Geometry check sheet. Reference: the model listing, model coordinates, mm. A direction names the side the tool comes from. Give positions to 0.01 mm unless a question says otherwise; leave off trailing zeros. Loops run counter-clockwise (first coordinate to the right, second up) from the corner with the lowest first, then second, coordinate; pieces in that order, holes last.
1. Go/stop test with flat-tipped pins: pin 1 Ø3 at (x, z) = (-36.5, 41) entering from -Y; pin 2 Ø10 at (y, z) = (23.5, 9) entering from -X; pin 3 Ø5.5 at (x, y) = (-39.5, 32) entering from +Z; pin 4 Ø2.5 at (x, z) = (39.5, 3.5) entering from +Y. Record where each tip stops, or that it passes through.
2. Cross-section at B-B, the plane y = 28. Record the cut outline in (x, z), plus the area to 3 significant figures.
3. Cross-section at C-C, the plane x = -20. Record the cut outline in (y, z).
4. Tool access check on faces 1 (the flat face through (-41.2, 22.3, 5)), 2 (the flat face through (0, 17, 5)), 3 (the flat face through (-43, 26, 25)), 4 (the flat face through (-39, 14.731, 25)). Record the directions out of +Z, -Z, +X, -X, +Y, -Y that give a thin tool (end or side, any length) a straight path to the whole face; none if there is none.
5. Release check for a two-part mould opening along Z. For faces 5 (the flat face through (-41.2, 25.6, 15)), 6 (the flat face through (0, 26, 50)), 7 (the flat face through (41, 29, 2)), 8 (the flat face through (0, 17, 0)) record: +Z half, -Z half, draft (parallel to the pull), parting line (faces both ways), or undercut.
6. Cross-section at D-D, the plane z = 3. Record the cut outline in (x, y), plus the area to 3 significant figures.
7. Material ranges on L1, parallel to Z at x = -36.5, y = 12.3; L2, parallel to X at y = 21, z = 3; L3, parallel to Z at x = -42, y = 29, recorded low to high.
8. Cross-section at A-A, the plane z = 25. Record the cut outline in (x, y).
from build123d import *

# Parameters (mm, degrees)
F1_DEPTH    = 50
F3_DEPTH    = 15
F5_DEPTH    = 15
F6_R        = 2.5
F7_DEPTH    = 93.001
F8_T1_DEPTH = 57.6539038248
F9_DEPTH    = 5
F10_R       = 2
F11_DEPTH   = 33


# Not quite as in the source:
# - a fillet or chamfer that OpenCascade refuses, or shapes differently, is made with other operations: its cross-section is extruded or revolved along the edge and cut away or added


with BuildPart() as f1:
    # F0 (on Top) → F1 (new body)
    with BuildSketch(Plane.XY):
        with BuildLine():
            ThreePointArc((-43, 8.7560448021), (-46.7056429154, 4.5424231597), (-50, 0))
            Line((-50, 0), (-47.5900705485, 0))
            ThreePointArc((-47.5900705485, 0), (-26.8784989109, 18.3696900801), (0, 25))
            ThreePointArc((0, 25), (26.8784989109, 18.3696900801), (47.5900705485, 0))
            Line((47.5900705485, 0), (50, 0))
            ThreePointArc((50, 0), (46.7056429154, 4.5424231597), (43, 8.7560448021))
            Line((43, 8.7560448021), (43, 43))
            Line((43, 43), (41, 43))
            Line((41, 43), (41, 14.7306729384))
            Line((41, 14.7306729384), (36.2875219066, 14.7306729384))
            ThreePointArc((36.2875219066, 14.7306729384), (0, 27), (-36.2875219066, 14.7306729384))
            Line((-36.2875219066, 14.7306729384), (-41, 14.7306729384))
            Line((-41, 14.7306729384), (-41, 43))
            Line((-41, 43), (-43, 43))
            Line((-43, 43), (-43, 8.7560448021))
        make_face()
    extrude(amount=F1_DEPTH)

    # F2 (on face) → F3 (cut)
    with BuildSketch(Plane.XY.offset(50)):
        Polygon((-43, 8.7560448021), (-36.2875219066, 14.7306729384), (-41, 14.7306729384), (-41, 43), (-43, 43), align=None)
        Polygon((41, 43), (41, 14.7306729384), (36.2875219066, 14.7306729384), (43, 8.7560448021), (43, 43), align=None)
    extrude(amount=-F3_DEPTH, mode=Mode.SUBTRACT)

    # F4 (on face) → F5 (cut)
    with BuildSketch(Plane(origin=(0, 0, 0), x_dir=(1, 0, 0), z_dir=(0, 0, -1))):
        Polygon((-36.2875219066, -14.7306729384), (-43, -8.7560448021), (-43, -43), (-41, -43), (-41, -14.7306729384), align=None)
        Polygon((43, -8.7560448021), (36.2875219066, -14.7306729384), (41, -14.7306729384), (41, -43), (43, -43), align=None)
    extrude(amount=-F5_DEPTH, mode=Mode.SUBTRACT)

    # F6 (on face) → F7 (cut, through all)
    with BuildSketch(Plane(origin=(-43, 0, 0), x_dir=(0, -1, 0), z_dir=(-1, 0, 0))):
        with Locations((-29.5, 25)):
            Circle(F6_R)
    extrude(amount=-F7_DEPTH, mode=Mode.SUBTRACT)

    # F8: chamfer of 1.5 on 2 edges, made by hand

    # F8_s2 → F8_t1 (cut)
    with BuildSketch(Plane.XY.offset(-3.8269519124)):
        with BuildLine():
            Line((-49.1206089535, -0.027238599), (-46.7036689522, 1.2042065191))
            Line((-46.7036689522, 1.2042065191), (-46.6793989906, 1.186572207))
            ThreePointArc((-46.6793989906, 1.186572207), (-47.1374385844, 0.5954223102), (-47.565368237, -0.0170233899))
            Line((-47.565368237, -0.0170233899), (-47.5900705485, -0.03))
            ThreePointArc((-47.5900705485, -0.03), (-48.355339751, -0.03), (-49.1206089535, -0.057238599))
            Line((-49.1206089535, -0.057238599), (-49.1206089535, -0.027238599))
        make_face()
        with BuildLine():
            Line((46.7036689522, 1.2042065191), (49.1206089535, -0.027238599))
            Line((49.1206089535, -0.027238599), (49.1206089535, -0.057238599))
            ThreePointArc((49.1206089535, -0.057238599), (48.355339751, -0.03), (47.5900705485, -0.03))
            Line((47.5900705485, -0.03), (47.565368237, -0.0170233899))
            ThreePointArc((47.565368237, -0.0170233899), (47.1374385844, 0.5954223102), (46.6793989906, 1.186572207))
            Line((46.6793989906, 1.186572207), (46.7036689522, 1.2042065191))
        make_face()
    extrude(amount=F8_T1_DEPTH, mode=Mode.SUBTRACT)

    # F0 (on Top) → F9 (join)
    with BuildSketch(Plane.XY):
        with BuildLine():
            ThreePointArc((-43, 8.7560448021), (-46.7056429154, 4.5424231597), (-50, 0))
            Line((-50, 0), (-47.5900705485, 0))
            ThreePointArc((-47.5900705485, 0), (-26.8784989109, 18.3696900801), (0, 25))
            ThreePointArc((0, 25), (26.8784989109, 18.3696900801), (47.5900705485, 0))
            Line((47.5900705485, 0), (50, 0))
            ThreePointArc((50, 0), (46.7056429154, 4.5424231597), (43, 8.7560448021))
            Line((43, 8.7560448021), (43, 43))
            Line((43, 43), (41, 43))
            Line((41, 43), (41, 14.7306729384))
            Line((41, 14.7306729384), (36.2875219066, 14.7306729384))
            ThreePointArc((36.2875219066, 14.7306729384), (0, 27), (-36.2875219066, 14.7306729384))
            Line((-36.2875219066, 14.7306729384), (-41, 14.7306729384))
            Line((-41, 14.7306729384), (-41, 43))
            Line((-41, 43), (-43, 43))
            Line((-43, 43), (-43, 8.7560448021))
        make_face()
        with BuildLine():
            ThreePointArc((0, 25), (-26.8784989109, 18.3696900801), (-47.5900705485, 0))
            Line((-47.5900705485, 0), (-37.5900705485, 0))
            ThreePointArc((-37.5900705485, 0), (-20.2249265861, 11.0833143525), (0, 15))
            Line((0, 15), (0, 25))
        make_face()
        with BuildLine():
            ThreePointArc((47.5900705485, 0), (26.8784989109, 18.3696900801), (0, 25))
            Line((0, 25), (0, 15))
            ThreePointArc((0, 15), (20.2249265861, 11.0833143525), (37.5900705485, 0))
            Line((37.5900705485, 0), (47.5900705485, 0))
        make_face()
    extrude(amount=F9_DEPTH)

    # F10 (on Front) → F11 (cut)
    with BuildSketch(Plane.XZ):
        with Locations((-36.5, 41)):
            Circle(F10_R)
        with Locations((-20, 41)):
            Circle(F10_R)
        with Locations((20, 41)):
            Circle(F10_R)
        with Locations((36.5, 41)):
            Circle(F10_R)
    extrude(amount=-F11_DEPTH, mode=Mode.SUBTRACT)


solid = f1.part
Result:
1. pin 1: passes through
1. pin 2: stops at x = -43
1. pin 3: stops at z = 35
1. pin 4: stops at y = 14.73
2. outline: (-43, 0) - (-41, 0) - (-41, 5) - (-43, 5) - close; (-43, 15) - (-41, 15) - (-41, 23) - (-43, 23) - close; (-43, 27) - (-41, 27) - (-41, 35) - (-43, 35) - close; (41, 0) - (43, 0) - (43, 5) - (41, 5) - close; (41, 15) - (43, 15) - (43, 23) - (41, 23) - close; (41, 27) - (43, 27) - (43, 35) - (41, 35) - close
2. area: 84.0 mm2
3. outline: (11.17, 0) - (23.56, 0) - (23.56, 39) - (21.43, 39) - (21.43, 5) - (11.17, 5) - close; (21.43, 43) - (23.56, 43) - (23.56, 50) - (21.43, 50) - close
4. face 1: -X, +Y
4. face 2: +Z, -Y
4. face 3: +Z, -Z, -X, +Y
4. face 4: +Z, -Z, +Y
5. face 5: undercut
5. face 6: +Z half
5. face 7: draft
5. face 8: -Z half
6. outline: (-50, 0) - (-37.59, 0) arc R55 cw to (0, 15) arc R55 cw to (37.59, 0) - (50, 0) arc R59.8 ccw to (43, 8.76) - (43, 43) - (41, 43) - (41, 14.73) - (36.29, 14.73) arc R59.8 ccw to (-36.29, 14.73) - (-41, 14.73) - (-41, 43) - (-43, 43) - (-43, 8.76) arc R59.8 ccw to start
6. area: 1,280 mm2
7. L1: z = 0 to 39, 43 to 50
7. L2: x = -43 to -41, -26.11 to 26.11, 41 to 43
7. L3: z = 0 to 5, 15 to 22.55, 27.45 to 35
8. outline: (-50, 0) - (-49.07, 0) - (-46.76, 1.18) arc R57.8 cw to (46.76, 1.18) - (49.07, 0) - (50, 0) arc R59.8 ccw to (43, 8.76) - (43, 27) - (41, 27) - (41, 14.73) - (36.29, 14.73) arc R59.8 ccw to (-36.29, 14.73) - (-41, 14.73) - (-41, 27) - (-43, 27) - (-43, 8.76) arc R59.8 ccw to start; (-43, 32) - (-41, 32) - (-41, 43) - (-43, 43) - close; (41, 32) - (43, 32) - (43, 43) - (41, 43) - close
